Design review of the part built by this model. Coordinates are the model's own, in mm. Face numbers are marked on the shaded views. A direction names the side the tool comes from. Give positions to 0.01 mm unless a question says otherwise; leave off trailing zeros. Loops run counter-clockwise (first coordinate to the right, second up) from the corner with the lowest first, then second, coordinate; pieces in that order, holes last. Notation, with made-up numbers: (71, 79.25) -> (119, 79.25) arc R29 ccw to (119, 100.25) -> close; hole circle Ø7 at (48.25, 66.5). An arc over 180 degrees is marked (long way). Answer in a Markdown table with one row per item. Add a question column.
(1) For the marked faces 4, 5 and 6, list the 3-axis set-ups (+Z, -Z, +X, -X, +Y, -Y) from which the entire face can be reached by the end or side of a thin tool; tool diameter is ignored.
(2) For pin 1 (5 mm diameter, centred on x = 7.79, y = 56.05, fed in from +Z); pin 2 (1.5 mm diameter, centred on x = -8, y = 38, fed in from +Z); pin 3 (5.5 mm diameter, centred on x = -3.5, z = -17.5, fed in from +Y), all flat-tipped, find the tip position at first contact; note any pin that passes through.
(3) Draft analysis for pull direction Z (two halves, no side actions). For the marked faces 1, 2 and 3, state which applies: +Z half, -Z half, draft (parallel to the pull), parting line (faces both ways), or undercut.
(4) Consider section D-D on z = 22.5. Write out the cut boundary in (x, y), then the cut area to 3 significant figures.
(5) Consider section C-C on y = 6.55. Write out the cut boundary in (x, z).
(6) For line 1 (X direction, y = -8, z = 28.5); line 2 (X direction, y = 56, z = -9); line 3 (X direction, y = 22, z = 2.5), list the stretches that pass through material, from the lowest coordinate up.
(7) Consider section B-B on y = 56.05. Write out the cut boundary in (x, z).
(8) Consider section A-A on z = 11.5. Write out the cut boundary in (x, y).
from build123d import *

# Parameters (mm, degrees)
SKETCH1_W               = 25
SKETCH1_H               = 17
BOSS_EXTRUDE1_DEPTH     = 12
MOVE_FACE1_BY           = 15
MOVE_FACE3_BY           = 8
SKETCH3_W               = 25
SKETCH3_H               = 12.751689795
BOSS_EXTRUDE2_DEPTH     = 6.9
SKETCH4_W               = 5
SKETCH4_H               = 16.698310205
BOSS_EXTRUDE3_DEPTH     = 6.9
MOVE_START              = -11.609792285
MOVE_FACE4_OUTLINE_W    = 6.9
MOVE_FACE4_OUTLINE_H    = 16.698310205
MOVE_FACE4_DEPTH        = 2.4
MOVE_FACE5_BY           = 20
SKETCH6_W               = 25
SKETCH6_H               = 10.9
BOSS_EXTRUDE5_DEPTH     = 2
MOVE_FACE6_BY           = 1.5
MOVE_FACE7_BY           = 2.6
SKETCH7_W               = 3.8
SKETCH7_H               = 30.95
BOSS_EXTRUDE6_DEPTH     = 41
SKETCH8_W               = 16.2
SKETCH8_H               = 3.5
BOSS_EXTRUDE7_DEPTH     = 41
SKETCH9_W               = 3
SKETCH9_H               = 30.95
BOSS_EXTRUDE8_DEPTH     = 41
SKETCH10_W              = 4.6
SKETCH10_H              = 3.5
BOSS_EXTRUDE9_DEPTH     = 41
MOVE_FACE8_BY           = 9
MOVE_FACE9_OUTLINE_W    = 6
MOVE_FACE9_OUTLINE_H    = 6.301689795
MOVE_FACE9_OUTLINE_H_2  = 3.5
MOVE_FACE9_DEPTH        = 27.6
MOVE_START_2            = 8.390207715
MOVE_FACE9_2_OUTLINE_W  = 6
MOVE_FACE9_2_OUTLINE_H  = 23.698310205
MOVE_FACE9_2_DEPTH      = 7.6
MOVE_FACE9_3_OUTLINE_W  = 6
MOVE_FACE9_3_OUTLINE_H  = 23.698310205
MOVE_FACE9_3_DEPTH      = 7.4
MOVE_FACE10_BY          = 10
SKETCH11_W              = 27.6
SKETCH11_H              = 3
BOSS_EXTRUDE10_DEPTH    = 11
SKETCH12_R              = 1.5
CUT_EXTRUDE1_DEPTH      = 16
SKETCH13_R              = 1.6
CUT_EXTRUDE2_DEPTH      = 5
SKETCH14_R              = 1.6
CUT_EXTRUDE3_DEPTH      = 9
SKETCH15_R              = 1.6
CUT_EXTRUDE4_DEPTH      = 5
MOVE_FACE14_BY          = 1
MOVE_FACE15_OUTLINE_W   = 16.9
MOVE_FACE15_OUTLINE_H   = 23.698310205
MOVE_FACE15_DEPTH       = 2
MOVE_FACE16_BY          = 8
MOVE_FACE17_BY          = 6
MOVE_FACE19_BY          = 6
MOVE_FACE20_BY          = 5
MOVE_FACE21_BY          = 0.2
MOVE_FACE22_BY          = 0.2
MOVE_START_3            = -12.454005935
MOVE_FACE23_OUTLINE_W   = 27.6
MOVE_FACE23_OUTLINE_H   = 62.9
MOVE_FACE23_DEPTH       = 0.05
MOVE_FACE24_BY          = 0.05
SKETCH17_R              = 1.6
CUT_EXTRUDE5_DEPTH      = 7.5
BOSS_EXTRUDE12_DEPTH    = 2
BOSS_EXTRUDE13_DEPTH    = 46
CUT_EXTRUDE6_DEPTH      = 70.24755409
CUT_EXTRUDE6_DEPTH_BACK = 70.24755409


# Read off the part's stored shape, not the designer's step: Move Face4, Move Face9, Move Face15, Move Face23
with BuildPart() as part:
    # Sketch1 → Boss-Extrude1 (new body)
    with BuildSketch(Plane(origin=(0, 0, 0), x_dir=(1, 0, 0), z_dir=(0, 1, 0))):
        with Locations((0.890207715, 2.454005935)):
            Rectangle(SKETCH1_W, SKETCH1_H)
    extrude(amount=BOSS_EXTRUDE1_DEPTH)

    # Move Face1: a face moved outward by 15.0
    extrude(part.faces().sort_by_distance((0.890207715, 6, 6.045994065))[0], amount=MOVE_FACE1_BY, dir=(0, 0, 1))

    # Move Face3: a face moved inward by 8.0
    extrude(part.faces().sort_by_distance((0.890207715, 12, 5.045994065))[0], amount=MOVE_FACE3_BY, dir=(0, -1, 0), mode=Mode.SUBTRACT)

    # Sketch3 → Boss-Extrude2 (add)
    with BuildSketch(Plane(origin=(0, 4, 0), x_dir=(1, 0, 0), z_dir=(0, 1, 0))):
        with Locations((0.890207715, -12.120149168)):
            Rectangle(SKETCH3_W, SKETCH3_H)
    extrude(amount=BOSS_EXTRUDE2_DEPTH)

    # Sketch4 → Boss-Extrude3 (add)
    with BuildSketch(Plane(origin=(0, 4, 0), x_dir=(1, 0, 0), z_dir=(0, 1, 0))):
        with Locations((10.890207715, 2.604850833)):
            Rectangle(SKETCH4_W, SKETCH4_H)
        with Locations((-6.709792285, 2.604850833)):
            Rectangle(SKETCH4_W, SKETCH4_H)
    extrude(amount=BOSS_EXTRUDE3_DEPTH)

    # Move Face4 outline → Move Face4 (add)
    with BuildSketch(Plane.YZ.offset(MOVE_START)):
        with Locations((7.45, -2.604850833)):
            Rectangle(MOVE_FACE4_OUTLINE_W, MOVE_FACE4_OUTLINE_H)
    extrude(amount=MOVE_FACE4_DEPTH)

    # Move Face5: a face moved inward by 20.0
    extrude(part.faces().sort_by_distance((2.090207715, 4, -2.604850832))[0], amount=MOVE_FACE5_BY, dir=(0, -1, 0), mode=Mode.SUBTRACT)

    # Sketch6 → Boss-Extrude5 (add)
    with BuildSketch(Plane(origin=(0, 0, -10.954005935), x_dir=(-1, 0, 0), z_dir=(0, 0, -1))):
        with Locations((-0.890207715, 5.45)):
            Rectangle(SKETCH6_W, SKETCH6_H)
    extrude(amount=-BOSS_EXTRUDE5_DEPTH)

    # Move Face6: a face moved outward by 1.5
    extrude(part.faces().sort_by_distance((0.890207715, 5.45, -10.954005935))[0], amount=MOVE_FACE6_BY, dir=(0, 0, -1))

    # Move Face7: a face moved outward by 2.6
    extrude(part.faces().sort_by_distance((13.390207715, 5.348749838, 3.512570938))[0], amount=MOVE_FACE7_BY, dir=(1, 0, 0))

    # Sketch7 → Boss-Extrude6 (add)
    with BuildSketch(Plane(origin=(0, 10.9, 0), x_dir=(1, 0, 0), z_dir=(0, 1, 0))):
        with Locations((-9.709792285, -3.020994065)):
            Rectangle(SKETCH7_W, SKETCH7_H)
    extrude(amount=BOSS_EXTRUDE6_DEPTH)

    # Sketch8 → Boss-Extrude7 (add)
    with BuildSketch(Plane(origin=(0, 10.9, 0), x_dir=(1, 0, 0), z_dir=(0, 1, 0))):
        with Locations((0.290207715, 10.704005935)):
            Rectangle(SKETCH8_W, SKETCH8_H)
    extrude(amount=BOSS_EXTRUDE7_DEPTH)

    # Sketch9 → Boss-Extrude8 (add)
    with BuildSketch(Plane(origin=(0, 10.9, 0), x_dir=(1, 0, 0), z_dir=(0, 1, 0))):
        with Locations((14.490207715, -3.020994065)):
            Rectangle(SKETCH9_W, SKETCH9_H)
    extrude(amount=BOSS_EXTRUDE8_DEPTH)

    # Sketch10 → Boss-Extrude9 (add)
    with BuildSketch(Plane(origin=(0, 10.9, 0), x_dir=(1, 0, 0), z_dir=(0, 1, 0))):
        with Locations((10.690207715, 10.704005935)):
            Rectangle(SKETCH10_W, SKETCH10_H)
    extrude(amount=BOSS_EXTRUDE9_DEPTH)

    # Move Face8: a face moved inward by 9.0
    extrude(part.faces().sort_by_distance((2.090207715, 5.45, 5.74430427))[0], amount=MOVE_FACE8_BY, dir=(0, 0, 1), mode=Mode.SUBTRACT)

    # Move Face9 outline → Move Face9 (add)
    with BuildSketch(Plane.YZ.offset(MOVE_START)):
        with Locations((-3, 17.895149168)):
            Rectangle(MOVE_FACE9_OUTLINE_W, MOVE_FACE9_OUTLINE_H)
        with Locations((-3, -10.704005935)):
            Rectangle(MOVE_FACE9_OUTLINE_W, MOVE_FACE9_OUTLINE_H_2)
    extrude(amount=MOVE_FACE9_DEPTH)

    # Move Face9 2 outline → Move Face9 2 (add)
    with BuildSketch(Plane.YZ.offset(MOVE_START_2)):
        with Locations((-3, 2.895149167)):
            Rectangle(MOVE_FACE9_2_OUTLINE_W, MOVE_FACE9_2_OUTLINE_H)
    extrude(amount=MOVE_FACE9_2_DEPTH)

    # Move Face9 3 outline → Move Face9 3 (add)
    with BuildSketch(Plane.YZ.offset(MOVE_START)):
        with Locations((-3, 2.895149167)):
            Rectangle(MOVE_FACE9_3_OUTLINE_W, MOVE_FACE9_3_OUTLINE_H)
    extrude(amount=MOVE_FACE9_3_DEPTH)

    # Move Face10: a face moved outward by 10.0
    extrude(part.faces().sort_by_distance((2.190207715, -1, 21.045994065))[0], amount=MOVE_FACE10_BY, dir=(0, 0, 1))

    # Sketch11 → Boss-Extrude10 (add)
    with BuildSketch(Plane(origin=(0, 0, -12.454005935), x_dir=(-1, 0, 0), z_dir=(0, 0, -1))):
        with Locations((-2.190207715, -4.5)):
            Rectangle(SKETCH11_W, SKETCH11_H)
    extrude(amount=BOSS_EXTRUDE10_DEPTH)

    # Sketch12 → Cut-Extrude1 (cut)
    with BuildSketch(Plane.XZ.offset(6)):
        with Locations(Location((-5.378312816, -20.454005935, 0), (0, 0, 270))):
            Circle(SKETCH12_R)
        with BuildLine():
            Line((-3.715791402, 28.545994065), (-3.715791402, 31.045994065))
            Line((-3.715791402, 31.045994065), (-7.07410382, 31.045994065))
            Line((-7.07410382, 31.045994065), (-7.115791402, 28.545994065))
            ThreePointArc((-7.115791402, 28.545994065), (-5.415791402, 26.845994065), (-3.715791402, 28.545994065))
        make_face()
    extrude(amount=-CUT_EXTRUDE1_DEPTH, mode=Mode.SUBTRACT)

    # Sketch13 → Cut-Extrude2 (cut)
    with BuildSketch(Plane(origin=(0, -3, 0), x_dir=(1, 0, 0), z_dir=(0, 1, 0))):
        with Locations(Location((9.990207715, 18.954005935, 0), (0, 0, 180))):
            Circle(SKETCH13_R)
        with BuildLine():
            Line((11.690207715, -27.045994065), (11.690207715, -31.045994065))
            Line((11.690207715, -31.045994065), (8.290207715, -31.045994065))
            Line((8.290207715, -31.045994065), (8.290207715, -27.045994065))
            ThreePointArc((8.290207715, -27.045994065), (9.990207715, -25.345994065), (11.690207715, -27.045994065))
        make_face()
    extrude(amount=-CUT_EXTRUDE2_DEPTH, mode=Mode.SUBTRACT)

    # Sketch14 → Cut-Extrude3 (cut)
    with BuildSketch(Plane.XZ.offset(3)):
        with Locations((9.990207715, 27.045994065)):
            Circle(SKETCH14_R)
    extrude(amount=-CUT_EXTRUDE3_DEPTH, mode=Mode.SUBTRACT)

    # Sketch15 → Cut-Extrude4 (cut)
    with BuildSketch(Plane.XY.offset(18.495994065)):
        with Locations((-2.209792285, 6.55)):
            Circle(SKETCH15_R)
        with Locations((7.790207715, 6.55)):
            Circle(SKETCH15_R)
    extrude(amount=-CUT_EXTRUDE4_DEPTH, mode=Mode.SUBTRACT)

    # Move Face14: a face moved inward by 1.0
    extrude(part.faces().sort_by_distance((-4.209792285, 2.45, 2.895149168))[0], amount=MOVE_FACE14_BY, dir=(-1, 0, 0), mode=Mode.SUBTRACT)

    # Move Face15 outline → Move Face15 (cut)
    with BuildSketch(Plane.YZ.offset(MOVE_START_2)):
        with Locations((2.45, 2.895149167)):
            Rectangle(MOVE_FACE15_OUTLINE_W, MOVE_FACE15_OUTLINE_H)
    extrude(amount=MOVE_FACE15_DEPTH, mode=Mode.SUBTRACT)

    # Move Face16: a face moved outward by 8.0
    extrude(part.faces().sort_by_distance((2.190207715, 51.9, -9.359005935))[0], amount=MOVE_FACE16_BY, dir=(0, 1, 0))

    # Move Face17: a face moved inward by 6.0
    extrude(part.faces().sort_by_distance((2.300746103, 4, 24.541741789))[0], amount=MOVE_FACE17_BY, dir=(0, -1, 0), mode=Mode.SUBTRACT)

    # Move Face19: a face moved outward by 6.0
    extrude(part.faces().sort_by_distance((13.230207715, -6, 3.795994065))[0], amount=MOVE_FACE19_BY, dir=(0, -1, 0))

    # Move Face20: a face moved inward by 5.0
    extrude(part.faces().sort_by_distance((2.300746103, -2, 24.541741789))[0], amount=MOVE_FACE20_BY, dir=(0, -1, 0), mode=Mode.SUBTRACT)

    # Move Face21: a face moved outward by 0.2
    extrude(part.faces().sort_by_distance((-7.809792285, 35.4, 4.770994065))[0], amount=MOVE_FACE21_BY, dir=(1, 0, 0))

    # Move Face22: a face moved outward by 0.2
    extrude(part.faces().sort_by_distance((12.990207715, 35.4, 4.770994065))[0], amount=MOVE_FACE22_BY, dir=(-1, 0, 0))

    # Move Face23 outline → Move Face23 (cut)
    with BuildSketch(Plane.XY.offset(MOVE_START_3)):
        with Locations((2.190207715, 28.45)):
            Rectangle(MOVE_FACE23_OUTLINE_W, MOVE_FACE23_OUTLINE_H)
    extrude(amount=MOVE_FACE23_DEPTH, mode=Mode.SUBTRACT)

    # Move Face24: a face moved outward by 0.05
    extrude(part.faces().sort_by_distance((2.590207715, 25.934788184, -8.954005935))[0], amount=MOVE_FACE24_BY, dir=(0, 0, 1))

    # Sketch17 → Cut-Extrude5 (cut)
    with BuildSketch(Plane.XY.offset(-8.904005935)):
        with Locations((-2.209792285, 56.05)):
            Circle(SKETCH17_R)
        with Locations((7.790207715, 56.05)):
            Circle(SKETCH17_R)
    extrude(amount=-CUT_EXTRUDE5_DEPTH, mode=Mode.SUBTRACT)

    # Sketch19 → Boss-Extrude12 (add)
    with BuildSketch(Plane(origin=(3.990207715, 0, 0), x_dir=(0, 0, -1), z_dir=(1, 0, 0))):
        Polygon((23.454005935, -3), (12.404005935, 43), (12.404005935, -3), align=None)
    extrude(amount=-BOSS_EXTRUDE12_DEPTH)

    # Sketch20 → Boss-Extrude13 (add)
    with BuildSketch(Plane(origin=(0, -3, 0), x_dir=(1, 0, 0), z_dir=(0, 1, 0))):
        Polygon((1.990207715, 15.804005935), (-1.409792285, 12.404005935), (1.990207715, 12.404005935), align=None)
        Polygon((3.990207715, 15.804005935), (7.390207715, 12.404005935), (3.990207715, 12.404005935), align=None)
    extrude(amount=BOSS_EXTRUDE13_DEPTH)

    # Sketch21 → Cut-Extrude6 (cut, two sides: drawn at the far end of the back side and taken through both)
    with BuildSketch(Plane(origin=(3.990207715, 0, 0), x_dir=(0, 0, -1), z_dir=(1, 0, 0)).offset(-CUT_EXTRUDE6_DEPTH_BACK)):
        Polygon((15.902869946, 28.434593255), (12.404005935, 43), (16.038201458, 43), align=None)
    extrude(amount=CUT_EXTRUDE6_DEPTH + CUT_EXTRUDE6_DEPTH_BACK, mode=Mode.SUBTRACT)


solid = part.part
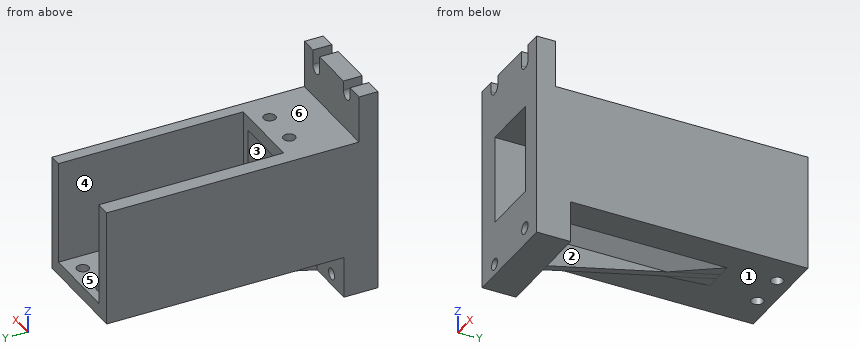
Values follow:
| question | item | result |
|---|---|---|
| 1 | face 4 | +Z, +Y |
| 1 | face 5 | +Y |
| 1 | face 6 | +Z, +X, -X, +Y |
| 2 | pin 1 | z = -8.9 |
| 2 | pin 2 | z = 18.5 |
| 2 | pin 3 | y = -3 |
| 3 | face 1 | -Z half |
| 3 | face 2 | draft |
| 3 | face 3 | undercut |
| 4 | outline | (-11.61, -12) -> (15.99, -12) -> (15.99, -7) -> (-11.61, -7) -> close |
| 4 | area | 138 mm2 |
| 5 | outline | (-11.61, -12.4) -> (-1.41, -12.4) -> (1.99, -15.8) -> (1.99, -21.16) -> (3.99, -21.16) -> (3.99, -15.8) -> (7.39, -12.4) -> (15.99, -12.4) -> (15.99, 18.5) -> (9.39, 18.5) -> (9.39, 14.74) -> (10.39, 14.74) -> (10.39, -8.9) -> (-5.21, -8.9) -> (-5.21, 14.74) -> (-3.81, 14.74) -> (-3.81, 18.5) -> (-11.61, 18.5) -> close; (-0.61, 14.74) -> (6.19, 14.74) -> (6.19, 18.5) -> (-0.61, 18.5) -> close |
| 6 | line 1 | -11.61 to -7.12, -3.72 to 8.29, 11.69 to 15.99 |
| 6 | line 2 | -11.61 to -3.81, -0.61 to 6.19, 9.39 to 15.99 |
| 6 | line 3 | -11.61 to -7.61, 12.79 to 15.99 |
| 7 | outline | (-11.61, -12.4) -> (-3.81, -12.4) -> (-3.81, -8.9) -> (-7.61, -8.9) -> (-7.61, 18.5) -> (-11.61, 18.5) -> close; (-0.61, -12.4) -> (6.19, -12.4) -> (6.19, -8.9) -> (-0.61, -8.9) -> close; (9.39, -12.4) -> (15.99, -12.4) -> (15.99, 18.5) -> (12.79, 18.5) -> (12.79, -8.9) -> (9.39, -8.9) -> close |
| 8 | outline | (-11.61, -12) -> (-5.21, -12) -> (-5.21, 10.9) -> (-7.61, 10.9) -> (-7.61, 59.9) -> (-11.61, 59.9) -> close; (10.39, -12) -> (15.99, -12) -> (15.99, 59.9) -> (12.79, 59.9) -> (12.79, 10.9) -> (10.39, 10.9) -> close |
